Check sheet for the modelled part. Datum: model origin and axes. Units: mm. Face numbers are marked on the shaded views. A direction names the side the tool comes from. Give positions to 0.01 mm unless a question says otherwise; leave off trailing zeros. Order: outer loops, then holes, each group sorted by start corner. A loop starts at its lowest first (then second) coordinate and runs counter-clockwise, first axis right, second up.
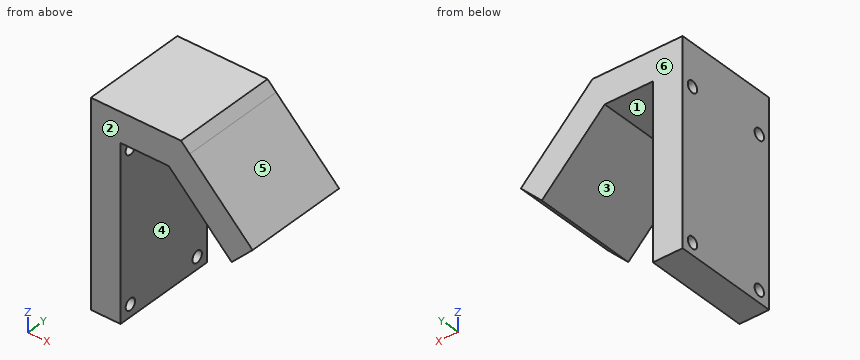
Solid Edge part; units mm, degrees
sketch "Sketch1" plane through (0, 0, 0) normal (1, 0, 0) x (0, 1, 0)
  line L0 (-14.25, -27.25) -> (-14.25, 27.25)
  line L1 (-14.25, 27.25) -> (14.25, 27.25)
  line L2 (14.25, 27.25) -> (14.25, -27.25)
  line L3 (14.25, -27.25) -> (-14.25, -27.25)
extrude "Protrusion1" add sketch "Sketch1" along normal blind 8
sketch "Sketch2" plane through (8, 0, 0) normal (1, 0, 0) x (0, 1, 0)
  line L0 (14.25, 19.25) -> (-14.25, 19.25)
  line L1 (-14.25, 19.25) -> (-14.25, 27.25)
  line L2 (-14.25, 27.25) -> (14.25, 27.25)
  line L3 (14.25, 27.25) -> (14.25, 19.25)
extrude "Extrusionsausprägung_2" add sketch "Sketch2" along normal blind 13
hole "Bohrung_1" at (0, 11, -24) direction (1, 0, 0) diameter 3.1 end through all
pattern_linear "Pattern1" count 2 spacing 22 along (0, -1, 0) count 2 spacing 40 along (0, 0, 1) of "Bohrung_1"
draft "Formschräge_3" angle 45 neutral plane through (18.75, 0, 19.25) normal (0, 0, -1) pull direction (0, 0, -1) face at (21, 9.215, 25.9967)
sketch "Sketch3" plane through (29.25, 0, 27.5) normal (0.7071068, 0, -0.7071068) x (0, 1, 0)
  line L0 (-14.25, -11.6673) -> (14.25, -11.6673)
  line L1 (14.25, -11.6673) -> (14.25, -3.6673)
  line L2 (14.25, -3.6673) -> (-14.25, -3.6673)
  line L3 (-14.25, -3.6673) -> (-14.25, -11.6673)
extrude "Extrusionsausprägung_3" add sketch "Sketch3" along normal blind 24
hole "Bohrung_3" [suppressed]
pattern "Pattern3" [suppressed]
sketch "Sketch4" plane through (32.5061, -14.25, 0) normal (0, -1, 0) x (1, 0, 0)
  line L0 (-5.8492, 24.9069) -> (-8.1924, 27.25)
extrude "Cutout1" cut sketch "Sketch4" against normal through all material side at (25.5207, -14.25, 26.1138)
1) Set-up check for the marked faces 1 and 2: record each of +Z, -Z, +X, -X, +Y, -Y from which the full face is reachable in a straight line by a thin tool's end or side.
Recorded:
face 1: -Z, +Y, -Y
face 2: +Z, -Z, +X, -X, -Y
2) Section check A-A, the plane z = -24. Record the cut outline in (x, y), then the cut area to 3 significant figures.
Recorded:
outline: (0, -14.25) - (8, -14.25) - (8, -12.55) - (0, -12.55) - close; (0, -9.45) - (8, -9.45) - (8, 9.45) - (0, 9.45) - close; (0, 12.55) - (8, 12.55) - (8, 14.25) - (0, 14.25) - close
area: 178 mm2
3) Section check D-D, the plane z = 16. Record the cut outline in (x, y).
Recorded:
outline: (0, -14.25) - (8, -14.25) - (8, -12.55) - (0, -12.55) - close; (0, -9.45) - (8, -9.45) - (8, 9.45) - (0, 9.45) - close; (0, 12.55) - (8, 12.55) - (8, 14.25) - (0, 14.25) - close; (24.25, -14.25) - (35.56, -14.25) - (35.56, 14.25) - (24.25, 14.25) - close
4) Material ranges on L1, parallel to Y at x = 5.25, z = 16; L2, parallel to Z at x = 4, y = -11; L3, parallel to Z at x = 9, y = 1, recorded low to high.
Recorded:
L1: y = -14.25 to -12.55, -9.45 to 9.45, 12.55 to 14.25
L2: z = -27.25 to -25.55, -22.45 to 14.45, 17.55 to 27.25
L3: z = 19.25 to 27.25
5) Depth check by flat-ended pin: pin 1 Ø6.5 at (x, y) = (17.5, 0.5) entering from -Z; pin 2 Ø2 at (y, z) = (-11, -21) entering from +X; pin 3 Ø12 at (x, z) = (34.5, -5) entering from -Y; pin 4 Ø1.5 at (x, y) = (35, -2.5) entering from +Z. Enter the tip coordinate at first touch or a pass-through.
Recorded:
pin 1: stops at z = 19.25
pin 2: stops at x = 8
pin 3: passes through
pin 4: stops at z = 17.31
6) Section check B-B, the plane x = 6.5. Record the cut outline in (y, z), then the cut area to 3 significant figures.
Recorded:
outline: (-14.25, -27.25) - (14.25, -27.25) - (14.25, 27.25) - (-14.25, 27.25) - close; hole circle Ø3.1 at (-11, -24); hole circle Ø3.1 at (-11, 16); hole circle Ø3.1 at (11, -24); hole circle Ø3.1 at (11, 16)
area: 1,520 mm2
7) Draft check along X on the marked faces 3, 4, 5 and 6. Enter one of: +X half, -X half, draft (parallel to the pull), parting line (faces both ways), or undercut.
Recorded:
face 3: undercut
face 4: undercut
face 5: +X half
face 6: draft
8) Section check C-C, the plane y = -11. State how many separate pieces and enclosed holes the cut face has, then the cut area to 3 significant figures.
Recorded:
separate pieces: 3
enclosed holes: 0
area: 709 mm2
